Work out the finished part from the listing and answer in its coordinate system (mm). A direction names the side the tool comes from. Round coordinates to 2 decimals unless told otherwise and drop trailing zeros. Write each loop counter-clockwise with the first axis right and the second up, starting at its lowest first coordinate (ties: lowest second). Pieces come first, ordered by that corner, then holes. Notation, with made-up numbers: (53, 48) - (75, 48) arc R30 ccw to (75, 72) - close; hole circle Ø7 at (-39.75, 29). An arc over 180 degrees is marked (long way). Write item = value, one per line. Start each with the question number.
from build123d import *

# Parameters (mm, degrees)
SKETCH1_W            = 25.4
SKETCH1_H            = 19.35
BOSS_EXTRUDE1_DEPTH  = 6
SKETCH2_W            = 1.11
SKETCH2_H            = 0.75
CUT_EXTRUDE3_DEPTH   = 24.910510241
LPATTERN2_COUNT      = 13
LPATTERN2_PITCH      = 2
FILLET1_R            = 0.15
M4_CLEARANCE_HOLE1_D = 4.5


with BuildPart() as part:
    # Sketch1 → Boss-Extrude1 (new body)
    with BuildSketch(Plane(origin=(0, 0, 0), x_dir=(1, 0, 0), z_dir=(0, 1, 0))):
        Rectangle(SKETCH1_W, SKETCH1_H)
    extrude(amount=BOSS_EXTRUDE1_DEPTH)

    # Sketch2 → Cut-Extrude3 (cut, through all)
    with BuildSketch(Plane.XY.offset(9.675)):
        with Locations((-12.145, 5.625)):
            Rectangle(SKETCH2_W, SKETCH2_H)
    cut_extrude3 = extrude(amount=-CUT_EXTRUDE3_DEPTH, mode=Mode.SUBTRACT)

    # LPattern2: Cut-Extrude3 ×13
    with Locations(*[(i * LPATTERN2_PITCH, 0, 0) for i in range(1, LPATTERN2_COUNT)]):
        add(cut_extrude3, mode=Mode.SUBTRACT)

    # Fillet1
    fillet1_edges = [part.edges().sort_by_distance(p)[0] for p in [
        (-6.7, 6, 0),
        (-5.59, 6, 0),
        (-4.7, 6, 0),
        (-3.59, 6, 0),
        (-2.7, 6, 0),
        (-1.59, 6, 0),
        (-0.7, 6, 0),
        (0.41, 6, 0),
        (1.3, 6, 0),
        (2.41, 6, 0),
        (3.3, 6, 0),
        (4.41, 6, 0),
        (5.3, 6, 0),
        (6.41, 6, 0),
        (7.3, 6, 0),
        (8.41, 6, 0),
        (9.3, 6, 0),
        (10.41, 6, 0),
        (11.3, 6, 0),
        (12.41, 6, 0),
        (-11.59, 6, 0),
        (-10.7, 6, 0),
        (-9.59, 6, 0),
        (-8.7, 6, 0),
        (-7.59, 6, 0),
    ]]
    fillet(fillet1_edges, radius=FILLET1_R)

    # M4 Clearance Hole1 (through all)
    with Locations(Plane(origin=(0, 0, 0), x_dir=(-1, 0, 0), z_dir=(0, -1, 0))):
        with Locations((0, 0)):
            Hole(M4_CLEARANCE_HOLE1_D / 2)


solid = part.part
1. This flat-tipped pin is pushed along its axis until it touches: pin 1 (0.6 mm diameter, centred on x = 0, z = 5.5, fed in from +Y). Where does it stop, or does it pass through?
2. Consider line 1 (Z direction, x = 0, y = 4) (3 decimals); line 2 (Y direction, x = 11.5, z = -1); line 3 (Z direction, x = -0.75, y = 0.75) (3 decimals). Determine where each line is inside the solid, lowest interval first.
3. Find section A-A on x = 0. Give the vertices of the cut face in (y, z) (3 decimals).
4. For a pull along X with two mould halves and no side action, classify faces 1 (the face through (-2.4, 5.25, 0.1)), 2 (the face through (-12, 5.25, 0)), 3 (the face through (-12.7, 3, 0)), 4 (the face through (6, 5.25, 0)) as released by +X, released by -X, zero draft, split by the parting line, or undercut.
5. Find section C-C on x = -6. Give the vertices of the cut face in (y, z) (3 decimals), plus the area to 3 significant figures.
6. Which of the six approach directions +Z, -Z, +X, -X, +Y, -Y give full straight-line access (tool end or side, diameter ignored) to faces 5 (the face through (0, 5.25, -6)), 6 (the face through (2.146, 3.042, -0.676))?
7. Find section B-B on y = 1.5. Give the vertices of the cut face in (x, z) (3 decimals).
Answer key:
q1.pin_1 = 5.25
q2.line_1 = -9.675 to -2.25, 2.25 to 9.675
q2.line_2 = 0 to 5.25
q2.line_3 = -9.675 to -2.121, 2.121 to 9.675
q3.outline = (0, -9.675) - (5.25, -9.675) - (5.25, -2.25) - (0, -2.25) - close; (0, 2.25) - (5.25, 2.25) - (5.25, 9.675) - (0, 9.675) - close
q4.face_1 = undercut
q4.face_2 = zero draft
q4.face_3 = released by -X
q4.face_4 = undercut
q5.outline = (0, -9.675) - (5.25, -9.675) - (5.25, 9.675) - (0, 9.675) - close
q5.area = 102 mm²
q6.face_5 = +Z, -Z, +Y
q6.face_6 = +Y, -Y
q7.outline = (-12.7, -9.675) - (12.7, -9.675) - (12.7, 9.675) - (-12.7, 9.675) - close; hole circle Ø4.5 at (0, 0)
